from build123d import *

# Parameters (mm, degrees)
F0_W     = 69
F0_H     = 115
F0_W_2   = 8.02
F0_H_2   = 8.02
F0_W_3   = 5
F0_H_3   = 2.2
F0_R     = 1.8
F1_DEPTH = 3


with BuildPart() as f1:
    # F0 (on Front) → F1 (new body)
    with BuildSketch(Plane.XZ):
        with Locations((34.5, 57.5)):
            Rectangle(F0_W, F0_H)
        with Locations((45.25, 86)):
            Rectangle(F0_W_2, F0_H_2, mode=Mode.SUBTRACT)
        with Locations((49.595, 79.13)):
            Rectangle(F0_W_3, F0_H_3, mode=Mode.SUBTRACT)
        with Locations((55.27, 86)):
            Rectangle(F0_W_2, F0_H_2, mode=Mode.SUBTRACT)
        with Locations((45.89, 94.0001)):
            Circle(F0_R, mode=Mode.SUBTRACT)
        with Locations((49.595, 102)):
            Rectangle(F0_W_3, F0_H_3, mode=Mode.SUBTRACT)
        with Locations((53.89, 94.0001)):
            Circle(F0_R, mode=Mode.SUBTRACT)
    extrude(amount=F1_DEPTH)


solid = f1.part
Design review of the part built by this model. Coordinates are the model's own, in mm. A direction names the side the tool comes from. Coordinates: 2 decimals unless noted, no trailing zeros. Loops run counter-clockwise (first coordinate to the right, second up) from the corner with the lowest first, then second, coordinate; pieces in that order, holes last.
Item 1: For faces 4 (the flat face through (52.095, -1, 79)), 5 (the flat face through (34, -3, 58)), list the 3-axis set-ups (+Z, -Z, +X, -X, +Y, -Y) from which the entire face can be reached by the end or side of a thin tool; tool diameter is ignored.
Completed:
face 4: +Y, -Y
face 5: +Z, -Z, +X, -X, -Y
Item 2: Add section C-C (y = -1.2). Write out the cut boundary in (x, z) (3 decimals).
Completed:
outline: (0, 0) - (69, 0) - (69, 115) - (0, 115) - close; hole (41.24, 81.99) - (49.26, 81.99) - (49.26, 90.01) - (41.24, 90.01) - close; hole circle Ø3.6 at (45.89, 94); hole (47.095, 78.03) - (52.095, 78.03) - (52.095, 80.23) - (47.095, 80.23) - close; hole (47.095, 100.9) - (52.095, 100.9) - (52.095, 103.1) - (47.095, 103.1) - close; hole (51.26, 81.99) - (59.28, 81.99) - (59.28, 90.01) - (51.26, 90.01) - close; hole circle Ø3.6 at (53.89, 94)
Item 3: Add section A-A (z = 86). Write out the cut boundary in (x, y).
Completed:
outline: (0, -3) - (41.24, -3) - (41.24, 0) - (0, 0) - close; (49.26, -3) - (51.26, -3) - (51.26, 0) - (49.26, 0) - close; (59.28, -3) - (69, -3) - (69, 0) - (59.28, 0) - close
Item 4: Wall thickness on L1, parallel to Z at x = 45.89, y = -0.95; L2, parallel to X at y = -1.9, z = 87; L3, parallel to Z at x = 56.5, y = -2: over which ranges is each line inside the solid? List them lowest first.
Completed:
L1: z = 0 to 81.99, 90.01 to 92.2, 95.8 to 115
L2: x = 0 to 41.24, 49.26 to 51.26, 59.28 to 69
L3: z = 0 to 81.99, 90.01 to 115
Item 5: Draft analysis for pull direction Z (two halves, no side actions). For faces 1 (the flat face through (34, -1, 0)), 2 (the flat face through (45, -1, 81.99)), 3 (the flat face through (34, 0, 58)), state which applies: pulls with the +Z half, pulls with the -Z half, needs draft (parallel to the pull), parting line crosses it, or undercut.
Completed:
face 1: pulls with the -Z half
face 2: undercut
face 3: needs draft
Item 6: Add section B-B (x = 45.89). Write out the cut boundary in (y, z).
Completed:
outline: (-3, 0) - (0, 0) - (0, 81.99) - (-3, 81.99) - close; (-3, 90.01) - (0, 90.01) - (0, 92.2) - (-3, 92.2) - close; (-3, 95.8) - (0, 95.8) - (0, 115) - (-3, 115) - close
